from build123d import *

# Parameters (mm, degrees)
F1_DEPTH = 25
F2_SIZE2 = 1.0392304845
F2_SIZE  = 0.6
F3_SIZE2 = 1.0392304845
F3_SIZE  = 0.6
F4_W     = 7
F4_H     = 9
F5_DEPTH = 1.5
F6_W     = 50
F6_H     = 9
F7_DEPTH = 1
F8_SIZE2 = 2.5980762114
F8_SIZE  = 1.5
F9_SIZE  = 1.5
F10_R    = 1


with BuildPart() as f1:
    # F0 (on Front) → F1 (new body, symmetric)
    with BuildSketch(Plane.XZ):
        Polygon((0.85, 2.5), (0.85, -2.5), (-0.85, -2.5), (-0.85, 2.5), (-3.35, 2.5), (-3.35, -6.5), (3.35, -6.5), (3.35, 2.5), align=None)
    extrude(amount=F1_DEPTH, both=True)

    # F2
    f2_edges = [f1.edges().sort_by_distance(p)[0] for p in [
        (-0.85, 0, 2.5),
    ]]
    f2_side = f1.faces().sort_by_distance((-2.1, 0, 2.5))[0]
    chamfer(f2_edges, length=F2_SIZE, length2=F2_SIZE2, reference=f2_side)

    # F3
    f3_edges = [f1.edges().sort_by_distance(p)[0] for p in [
        (0.85, 0, 2.5),
    ]]
    f3_side = f1.faces().sort_by_distance((2.1, 0, 2.5))[0]
    chamfer(f3_edges, length=F3_SIZE, length2=F3_SIZE2, reference=f3_side)

    # F4 (on face) → F5 (join)
    with BuildSketch(Plane.YZ.offset(3.35)):
        with Locations((-21.5, -2)):
            Rectangle(F4_W, F4_H)
        with Locations((21.5, -2)):
            Rectangle(F4_W, F4_H)
    extrude(amount=F5_DEPTH)

    # F6 (on face) → F7 (join)
    with BuildSketch(Plane(origin=(-3.35, 0, 0), x_dir=(0, -1, 0), z_dir=(-1, 0, 0))):
        with Locations((0, -2)):
            Rectangle(F6_W, F6_H)
    extrude(amount=F7_DEPTH)

    # F8
    f8_edges = [f1.edges().sort_by_distance(p)[0] for p in [
        (-4.35, 0, 2.5),
    ]]
    f8_side = f1.faces().sort_by_distance((-2.9, 0, 2.5))[0]
    chamfer(f8_edges, length=F8_SIZE, length2=F8_SIZE2, reference=f8_side)

    # F9
    f9_edges = [f1.edges().sort_by_distance(p)[0] for p in [
        (-4.35, -25, -3.299038),
        (-4.35, 25, -3.299038),
    ]]
    chamfer(f9_edges, length=F9_SIZE)

    # F10
    f10_edges = [f1.edges().sort_by_distance(p)[0] for p in [
        (-0.85, 0, 1.46077),
        (-1.45, 0, 2.5),
        (1.45, 0, 2.5),
        (0.85, 0, 1.46077),
    ]]
    fillet(f10_edges, radius=F10_R)


solid = f1.part
The listing builds one solid part. Answer for the finished solid, in the listing's coordinates (mm). A direction names the side the tool comes from. Give positions to 0.01 mm unless a question says otherwise; leave off trailing zeros. Loops run counter-clockwise (first coordinate to the right, second up) from the corner with the lowest first, then second, coordinate; pieces in that order, holes last.
Item 1: A cutting plane is placed at B-B (y = 20.5). Give the vertices of the cut face in (x, z).
Derived:
outline: (-4.35, -6.5) - (4.85, -6.5) - (4.85, 2.5) - (2.03, 2.5) arc R1 ccw to (1.16, 2) - (0.98, 1.69) arc R1 ccw to (0.85, 1.19) - (0.85, -2.5) - (-0.85, -2.5) - (-0.85, 1.19) arc R1 ccw to (-0.98, 1.69) - (-1.16, 2) arc R1 ccw to (-2.03, 2.5) - (-2.85, 2.5) - (-4.35, -0.1) - close
Item 2: Find the intervals of material crossed by line 1 along X through (y, z) = (19, -0.5); line 2 along X through (y, z) = (14, -0.5); line 3 along X through (y, z) = (6, -6), in increasing order.
Derived:
line 1: x = -4.35 to -0.85, 0.85 to 4.85
line 2: x = -4.35 to -0.85, 0.85 to 3.35
line 3: x = -4.35 to 3.35
Item 3: A tool of negligible diameter and unlimited length cuts with its end or side. For faces 1 (the flat face through (-3.6, 0.3, 1.2)), 2 (the flat face through (3.35, 0, -2)), 3 (the cylindrical face through (1.534, 0.35, 2.37)), from which of +Z, -Z, +X, -X, +Y, -Y can it reach the whole face along a straight path? Write none if from no direction.
Derived:
face 1: +Z, -X, +Y, -Y
face 2: +Z, -Z, +X
face 3: +Z, +Y, -Y
Item 4: A cutting plane is placed at D-D (x = 0). Give the vertices of the cut face in (y, z), then the cut area to 3 significant figures.
Derived:
outline: (-25, -6.5) - (25, -6.5) - (25, -2.5) - (-25, -2.5) - close
area: 200 mm2
Item 5: A cutting plane is placed at C-C (z = -4.25). Give the vertices of the cut face in (x, y), then the cut area to 3 significant figures.
Derived:
outline: (-4.35, -23.5) - (-2.85, -25) - (4.85, -25) - (4.85, -18) - (3.35, -18) - (3.35, 18) - (4.85, 18) - (4.85, 25) - (-2.85, 25) - (-4.35, 23.5) - close
area: 404 mm2
Item 6: A cutting plane is placed at A-A (z = -1.25). Give the vertices of the cut face in (x, y).
Derived:
outline: (-4.35, -23.5) - (-2.85, -25) - (-0.85, -25) - (-0.85, 25) - (-2.85, 25) - (-4.35, 23.5) - close; (0.85, -25) - (4.85, -25) - (4.85, -18) - (3.35, -18) - (3.35, 18) - (4.85, 18) - (4.85, 25) - (0.85, 25) - close
Item 7: Each of these flat-tipped pins is pushed along its axis until it touches: pin 1 Ø1 at (x, y) = (-3, -8) entering from +Z; pin 2 Ø1.1 at (y, z) = (-1.5, -1) entering from +X; pin 3 Ø1 at (x, y) = (0, 5) entering from +Z. Where does it stop, or does it pass through?
Derived:
pin 1: stops at z = 2.5
pin 2: stops at x = 3.35
pin 3: stops at z = -2.5
